```python
from build123d import *

# Parameters (mm, degrees)
BOSS_EXTRUDE1_DEPTH = 1.5
CUT_EXTRUDE1_DEPTH  = 75.863208587
SKETCH6_W           = 1.5
SKETCH6_H           = 12
SKETCH6_H_2         = 16.5
SKETCH6_H_3         = 1.5
SKETCH6_W_2         = 8.5
SKETCH6_W_3         = 30
CUT_EXTRUDE2_DEPTH  = 75.863208587


with BuildPart() as part:
    # Sketch2 → Boss-Extrude1 (new body)
    with BuildSketch(Plane(origin=(0, 0, 0), x_dir=(1, 0, 0), z_dir=(0, 1, 0))):
        Polygon((-70, 23.5), (-49, 23.5), (-49, 26.5), (-20, 26.5), (-20, 23.5), (20, 23.5), (20, 26.5), (49, 26.5), (49, 23.5), (70, 23.5), (70, -23.5), (-70, -23.5), align=None)
    extrude(amount=BOSS_EXTRUDE1_DEPTH)

    # Sketch5 → Cut-Extrude1 (cut, through all)
    with BuildSketch(Plane(origin=(0, 1.5, 0), x_dir=(1, 0, 0), z_dir=(0, 1, 0))):
        Polygon((-4.133974596, -11.5), (-6.732050808, -13), (-6.732050808, -16), (-4.133974596, -17.5), (-1.535898385, -16), (-1.535898385, -13), align=None)
        Polygon((-12.401923789, -11.5), (-15, -13), (-15, -16), (-12.401923789, -17.5), (-9.803847577, -16), (-9.803847577, -13), align=None)
        Polygon((4.133974596, -11.5), (1.535898385, -13), (1.535898385, -16), (4.133974596, -17.5), (6.732050808, -16), (6.732050808, -13), align=None)
        Polygon((12.401923789, -11.5), (9.803847577, -13), (9.803847577, -16), (12.401923789, -17.5), (15, -16), (15, -13), align=None)
        Polygon((-4.133974596, -3.5), (-6.732050808, -5), (-6.732050808, -8), (-4.133974596, -9.5), (-1.535898385, -8), (-1.535898385, -5), align=None)
        Polygon((4.133974596, -3.5), (1.535898385, -5), (1.535898385, -8), (4.133974596, -9.5), (6.732050808, -8), (6.732050808, -5), align=None)
        Polygon((12.401923789, -3.5), (9.803847577, -5), (9.803847577, -8), (12.401923789, -9.5), (15, -8), (15, -5), align=None)
        Polygon((-4.133974596, 4.5), (-6.732050808, 3), (-6.732050808, 0), (-4.133974596, -1.5), (-1.535898385, 0), (-1.535898385, 3), align=None)
        Polygon((4.133974596, 4.5), (1.535898385, 3), (1.535898385, 0), (4.133974596, -1.5), (6.732050808, 0), (6.732050808, 3), align=None)
        Polygon((12.401923789, 4.5), (9.803847577, 3), (9.803847577, 0), (12.401923789, -1.5), (15, 0), (15, 3), align=None)
        Polygon((-4.133974596, 12.5), (-6.732050808, 11), (-6.732050808, 8), (-4.133974596, 6.5), (-1.535898385, 8), (-1.535898385, 11), align=None)
        Polygon((4.133974596, 12.5), (1.535898385, 11), (1.535898385, 8), (4.133974596, 6.5), (6.732050808, 8), (6.732050808, 11), align=None)
        Polygon((12.401923789, 12.5), (9.803847577, 11), (9.803847577, 8), (12.401923789, 6.5), (15, 8), (15, 11), align=None)
        Polygon((-12.401923789, -3.5), (-15, -5), (-15, -8), (-12.401923789, -9.5), (-9.803847577, -8), (-9.803847577, -5), align=None)
        Polygon((-12.401923789, 4.5), (-15, 3), (-15, 0), (-12.401923789, -1.5), (-9.803847577, 0), (-9.803847577, 3), align=None)
        Polygon((-12.401923789, 12.5), (-15, 11), (-15, 8), (-12.401923789, 6.5), (-9.803847577, 8), (-9.803847577, 11), align=None)
    extrude(amount=-CUT_EXTRUDE1_DEPTH, mode=Mode.SUBTRACT)

    # Sketch6 → Cut-Extrude2 (cut, through all)
    with BuildSketch(Plane(origin=(0, 1.5, 0), x_dir=(1, 0, 0), z_dir=(0, 1, 0))):
        with Locations((69.25, 17.5)):
            Rectangle(SKETCH6_W, SKETCH6_H)
        with Locations((69.25, -13.75)):
            Rectangle(SKETCH6_W, SKETCH6_H_2)
        with Locations((69.25, -22.75)):
            Rectangle(SKETCH6_W, SKETCH6_H_3)
        with Locations((64.25, -22.75)):
            Rectangle(SKETCH6_W_2, SKETCH6_H_3)
        with Locations((25, -22.75)):
            Rectangle(SKETCH6_W_3, SKETCH6_H_3)
        with Locations((-25, -22.75)):
            Rectangle(SKETCH6_W_3, SKETCH6_H_3)
        with Locations((-69.25, 17.5)):
            Rectangle(SKETCH6_W, SKETCH6_H)
        with Locations((-69.25, -13.75)):
            Rectangle(SKETCH6_W, SKETCH6_H_2)
        with Locations((-69.25, -22.75)):
            Rectangle(SKETCH6_W, SKETCH6_H_3)
        with Locations((-64.25, -22.75)):
            Rectangle(SKETCH6_W_2, SKETCH6_H_3)
    extrude(amount=-CUT_EXTRUDE2_DEPTH, mode=Mode.SUBTRACT)


solid = part.part
```
Geometry: final body of the model. Coordinates: model frame, mm. Coordinates: 2 decimals unless noted, no trailing zeros. Write each loop counter-clockwise with the first axis right and the second up, starting at its lowest first coordinate (ties: lowest second). Pieces come first, ordered by that corner, then holes. Notation, with made-up numbers: M 30,27 L 38,27 A20 ccw 38,61 Z; hole C 11,42.5 d2. An arc over 180 degrees is marked long. Answer as CSV lines item,"result". Start each with the question number.
Q1. Line query: line 1 (X direction, y = 1.35, z = 7.5); line 2 (X direction, y = 0.65, z = -11); line 3 (Z direction, x = 14.5, y = 1.3). Output: solid intervals per line, ascending. Write a range as from..to.
Q2. Cut plane B-B on x = 30. Return the cut outline in (y, z).
Q3. Cut plane C-C on z = -20.5. Return the cut outline in (x, y), then the cut area to 4 significant figures.
Q4. Pin query (flat end, axial travel): P1, Ø0.8, axis at y = 0.5, z = 6.5, coming from the +X side; P2, Ø0.8, axis at y = 1, z = 14, coming from the -X side; P3, Ø0.8, axis at y = 1, z = 23, coming from the +X side. Return the tip coordinate at first contact, or that it passes through.
Q5. Cut plane A-A on y = 0.9. Count the separate pieces of the cut face and the enclosed holes in it, then the cut area to 3 significant figures.
Findings below:
1,line 1,"x = -68.5..-15, -9.8..-6.73, -1.54..1.54, 6.73..9.8, 15..68.5"
1,line 2,"x = -70..-15, -9.8..-6.73, -1.54..1.54, 6.73..9.8, 15..70"
1,line 3,"z = -23.5..-11.29, -7.71..-3.29, 0.29..4.71, 8.29..12.71, 16.29..22"
2,outline,"M 0,-26.5 L 1.5,-26.5 L 1.5,22 L 0,22 Z"
3,outline,"M -68.5,0 L 68.5,0 L 68.5,1.5 L -68.5,1.5 Z"
3,area,"205.5 mm2"
4,P1,"stops at x = 68.5"
4,P2,"stops at x = -68.5"
4,P3,"stops at x = 60"
5,separate pieces,"1"
5,enclosed holes,"16"
5,area,"6,170 mm2"
